Model file for the job. Use its own axes, mm. Coordinates: 2 decimals unless noted, no trailing zeros. Write each loop counter-clockwise with the first axis right and the second up, starting at its lowest first coordinate (ties: lowest second). Pieces come first, ordered by that corner, then holes. Notation, with made-up numbers: (-33, 20) - (18, 20) arc R16 ccw to (18, 33) - close; hole circle Ø7 at (40, 41.5). An arc over 180 degrees is marked (long way). Put each result on its own line as item: value. Start each with the question number.
1. Drop flat-ended pins along their axis: P1, Ø1, axis at x = 3.5, z = 8, coming from the +Y side; P2, Ø1, axis at y = -2.5, z = 9, coming from the -X side; P3, Ø4, axis at x = 9, z = 6.5, coming from the +Y side; P4, Ø10, axis at x = 17.5, y = 5.5, coming from the -Z side. Give the stop position or say it passes through.
2. Saw through at A-A, the plane x = 0. Write the cut outline in (y, z) (3 decimals), plus the area to 3 significant figures.
3. Drill centre lines: L1, parallel to X at y = -4, z = 9.5; L2, parallel to Y at x = -12.5, z = 3.75; L3, parallel to X at y = 2.5, z = 0.5. Where is each one in solid material? Low to high. Write a range as from..to.
4. Saw through at B-B, the plane y = 7. Write the cut outline in (x, z).
5. Saw through at D-D, the plane y = 31.5. Write the cut outline in (x, z).
6. Saw through at C-C, the plane z = 7.25. Write the cut outline in (x, y) (1 decimal), plus the area to 3 significant figures.
7. Pull direction Y, two halves, no side cores. Call faces 1 (the face through (10.6, 3.34, 5.07)), 2 (the face through (2.631, 41.475, 4.93)), 3 (the face through (0, 14, 10)): released by +Y, released by -Y, zero draft, split by the parting line, or undercut.
```python
from build123d import *

# Parameters (mm, degrees)
F2_DEPTH = 10
F0_R     = 11.115
F3_DEPTH = 12.5


with BuildPart() as f2:
    # F1 (on Top) → F2 (new body)
    with BuildSketch(Plane.XY):
        with BuildLine():
            ThreePointArc((-15.105416, 18.650104), (-0.219685, 23.998995), (14.76147, 18.923504))
            ThreePointArc((14.76147, 18.923504), (2.357081, 41.724676), (-21.59713, 51.722581))
            ThreePointArc((-21.59713, 51.722581), (-9.295213, 36.963934), (-15.105416, 18.650104))
        make_face()
        with BuildLine():
            ThreePointArc((-15.105416, 18.650104), (-10.331263, -21.662525), (24, 0))
            ThreePointArc((24, 0), (21.56705, 10.529119), (14.76147, 18.923504))
            ThreePointArc((14.76147, 18.923504), (-0.219685, 23.998995), (-15.105416, 18.650104))
        make_face()
    extrude(amount=F2_DEPTH)

    # F0 (on Top) → F3 (cut, symmetric)
    with BuildSketch(Plane.XY):
        Circle(F0_R)
    extrude(amount=F3_DEPTH, both=True, mode=Mode.SUBTRACT)


solid = f2.part
```
Final values:
1. P1: stops at y = 41.13
1. P2: stops at x = -23.92
1. P3: stops at y = 36.74
1. P4: stops at z = 0
2. outline: (-24, 0) - (-11.115, 0) - (-11.115, 10) - (-24, 10) - close; (11.115, 0) - (43.689, 0) - (43.689, 10) - (11.115, 10) - close
2. area: 455 mm²
3. L1: x = -23.66..-10.37, 10.37..23.66
3. L2: y = -20.49..21.69, 44.53..50.11
3. L3: x = -23.87..-10.83, 10.83..23.87
4. outline: (-22.96, 0) - (-8.63, 0) - (-8.63, 10) - (-22.96, 10) - close; (8.63, 0) - (22.96, 0) - (22.96, 10) - (8.63, 10) - close
5. outline: (-8.99, 0) - (10.44, 0) - (10.44, 10) - (-8.99, 10) - close
6. outline: (-21.6, 51.7) arc R20 cw to (-15.1, 18.7) arc R24 ccw (long way) to (24, 0) arc R24 ccw to (14.8, 18.9) arc R39.1 ccw to start; hole circle Ø22.2 at (0, 0)
6. area: 1,880 mm²
7. face 1: undercut
7. face 2: released by +Y
7. face 3: zero draft
